Source: CAD feature listing. Evaluate the final solid. Frame: model axes, mm. A direction names the side the tool comes from. Give positions to 0.01 mm unless a question says otherwise; leave off trailing zeros.
1) Access query for faces 1 (the face through (-1, 14, 48)), 2 (the face through (54.5, 9, 0)), 3 (the face through (-54.5, 4, 0)). Directions: +Z, -Z, +X, -X, +Y, -Y. A direction counts if a zero-diameter tool reaches every point of the face in a straight line with its end or side. Return the directions, or none.
2) Draft query along Y for faces 4 (the face through (-1, 16.5, 1)), 5 (the face through (-54.5, -4, 0)), 6 (the face through (-56.5, -6, -1)). Return one class per face: released by +Y, released by -Y, zero draft, split by the parting line, or undercut.
3) First-contact query: P1, Ø1.3, axis at x = -6, y = -8.5, coming from the +Z side; P2, Ø1.3, axis at y = -14.5, z = -12.5, coming from the +X side; P3, Ø0.8, axis at y = -13.5, z = 0.5, coming from the -X side. Flat tips, straight axial feed; report the tip coordinate or a pass-through.
4) Material intervals for line 1 (Z direction, x = -37.5, y = 9); line 2 (X direction, y = 8.5, z = -36.5), sorted ascending.
```python
from build123d import *

# Parameters (mm, degrees)
F0_W     = 113
F0_H     = 100
F1_DEPTH = 16.5
F2_W     = 113
F2_H     = 2.648482
F3_DEPTH = 2
F4_W     = 2.648482
F4_H     = 98
F5_DEPTH = 2
F6_W     = 2.648482
F6_H     = 98
F7_DEPTH = 2


with BuildPart() as f1:
    # F0 (on Front) → F1 (new body, symmetric)
    with BuildSketch(Plane.XZ):
        Rectangle(F0_W, F0_H)
    extrude(amount=F1_DEPTH, both=True)

    # F2 (on face) → F3 (cut)
    with BuildSketch(Plane.XY.offset(50)):
        with Locations((0, -14.097255)):
            Rectangle(F2_W, F2_H)
        with Locations((0, 14.097255)):
            Rectangle(F2_W, F2_H)
        with Locations((0, -9.271692)):
            Rectangle(F2_W, F2_H)
        with Locations((0, -3.639926)):
            Rectangle(F2_W, F2_H)
        with Locations((0, 3.639926)):
            Rectangle(F2_W, F2_H)
        with Locations((0, 9.271692)):
            Rectangle(F2_W, F2_H)
    extrude(amount=-F3_DEPTH, mode=Mode.SUBTRACT)

    # F4 (on face) → F5 (cut)
    with BuildSketch(Plane.YZ.offset(56.5)):
        with Locations((14.097255, -1)):
            Rectangle(F4_W, F4_H)
        with Locations((9.271692, -1)):
            Rectangle(F4_W, F4_H)
        with Locations((3.639926, -1)):
            Rectangle(F4_W, F4_H)
        with Locations((-3.639926, -1)):
            Rectangle(F4_W, F4_H)
        with Locations((-9.271692, -1)):
            Rectangle(F4_W, F4_H)
        with Locations((-14.097255, -1)):
            Rectangle(F4_W, F4_H)
    extrude(amount=-F5_DEPTH, mode=Mode.SUBTRACT)

    # F6 (on face) → F7 (cut)
    with BuildSketch(Plane(origin=(-56.5, 0, 0), x_dir=(0, -1, 0), z_dir=(-1, 0, 0))):
        with Locations((-14.097255, -1)):
            Rectangle(F6_W, F6_H)
        with Locations((-9.271692, -1)):
            Rectangle(F6_W, F6_H)
        with Locations((-3.639926, -1)):
            Rectangle(F6_W, F6_H)
        with Locations((3.639926, -1)):
            Rectangle(F6_W, F6_H)
        with Locations((9.271692, -1)):
            Rectangle(F6_W, F6_H)
        with Locations((14.097255, -1)):
            Rectangle(F6_W, F6_H)
    extrude(amount=-F7_DEPTH, mode=Mode.SUBTRACT)


solid = f1.part
```
From the geometry:
1. face 1: +Z, +X, -X
1. face 2: +Z, -Z, +X
1. face 3: +Z, -Z, -X
2. face 4: released by +Y
2. face 5: undercut
2. face 6: zero draft
3. P1: stops at z = 50
3. P2: stops at x = 54.5
3. P3: stops at x = -54.5
4. line 1: z = -50 to 48
4. line 2: x = -54.5 to 54.5
